Design review of the part shown in the three views and the two pictorial views. Dimensions are in mm from the part's minimum x, y and z. A direction names the side the tool comes from. Round coordinates to 2 decimals unless told otherwise and drop trailing zeros. Order: outer loops, then holes, each group sorted by start corner. A loop starts at its lowest first (then second) coordinate and runs counter-clockwise, first axis right, second up. Notation, with made-up numbers: M 27.5,15 L 35.5,15 A20 ccw 35.5,34 Z; hole C 84,-23 d7. An arc over 180 degrees is marked long. Write item = value, one per line. Start each with the question number.
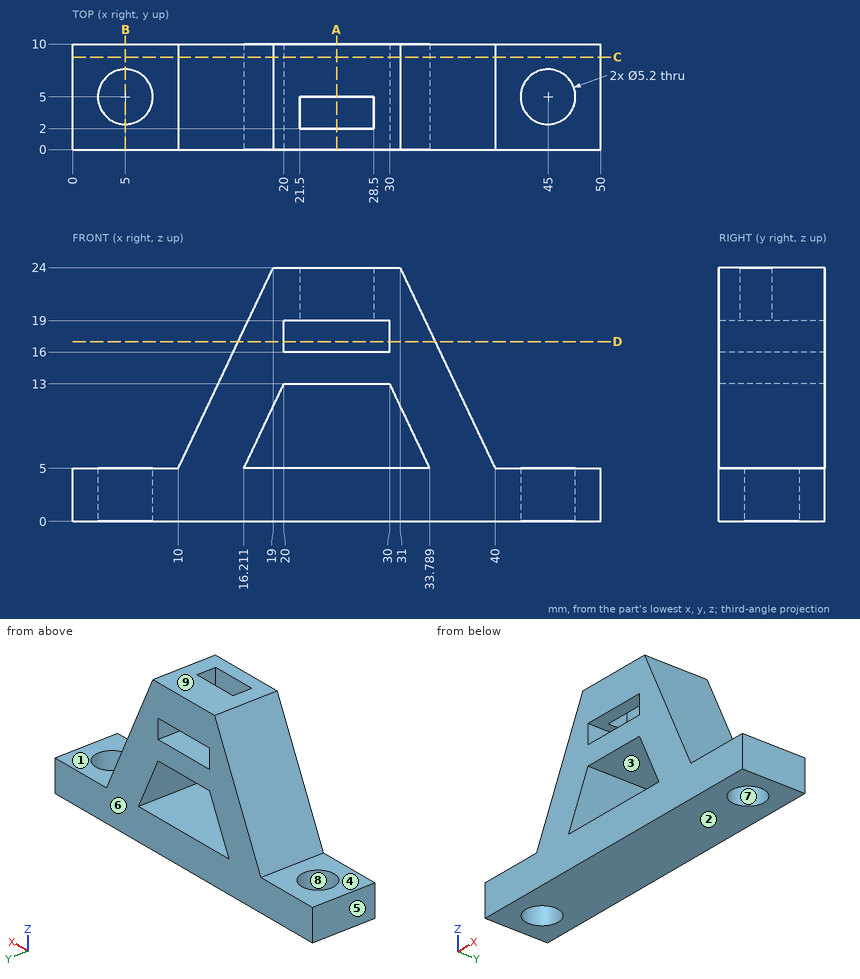
(1) Insertion check: pin 1 (1 mm diameter, centred on y = 3, z = 12.5, fed in from +X) (1 decimal); pin 2 (5 mm diameter, centred on x = 6, y = 5, fed in from +Z); pin 3 (1 mm diameter, centred on y = 4, z = 14.5, fed in from +X). Each pin has a flat end and moves straight along its axis. Give the tip position at first contact, or say it passes through.
(2) We need section C-C, the plane y = 8.75. Write out the cut boundary in (x, z).
(3) We need section B-B, the plane x = 5. Write out the cut boundary in (y, z).
(4) We need section D-D, the plane z = 17. Write out the cut boundary in (x, y) (1 decimal).
(5) We need section A-A, the plane x = 25. Write out the cut boundary in (y, z), then the cut area to 3 significant figures.
(6) Draft analysis for pull direction Y (two halves, no side actions). For the marked faces 6, 7, 8 and 9, state which applies: released by +Y, released by -Y, zero draft, split by the parting line, or undercut.
(7) For the marked faces 1, 2, 3, 4 and 5, list the 3-axis set-ups (+Z, -Z, +X, -X, +Y, -Y) from which the entire face can be reached by the end or side of a thin tool; tool diameter is ignored.
(8) For line 1 along Z through (x, y) = (21, 3.5); line 2 along Y through (x, z) = (5, 3.3); line 3 along Y through (x, z) = (23, 20), list the stretches that pass through material, from the lowest coordinate up.
Values:
q1.pin_1 = 36.7
q1.pin_2 = 5
q1.pin_3 = 35.74
q2.outline = M 0,0 L 50,0 L 50,5 L 40,5 L 31,24 L 19,24 L 10,5 L 0,5 Z; hole M 16.21,5 L 33.79,5 L 30,13 L 20,13 Z; hole M 20,16 L 30,16 L 30,19 L 20,19 Z
q3.outline = M 0,0 L 2.4,0 L 2.4,5 L 0,5 Z; M 7.6,0 L 10,0 L 10,5 L 7.6,5 Z
q4.outline = M 15.7,0 L 20,0 L 20,10 L 15.7,10 Z; M 30,0 L 34.3,0 L 34.3,10 L 30,10 Z
q5.outline = M 0,0 L 10,0 L 10,5 L 0,5 Z; M 0,13 L 10,13 L 10,16 L 0,16 Z; M 0,19 L 2,19 L 2,24 L 0,24 Z; M 5,19 L 10,19 L 10,24 L 5,24 Z
q5.area = 115 mm²
q6.face_6 = released by +Y
q6.face_7 = undercut
q6.face_8 = undercut
q6.face_9 = zero draft
q7.face_1 = +Z, +X, +Y, -Y
q7.face_2 = -Z, +X, -X, +Y, -Y
q7.face_3 = +Y, -Y
q7.face_4 = +Z, -X, +Y, -Y
q7.face_5 = +Z, -Z, -X, +Y, -Y
q8.line_1 = 0 to 5, 13 to 16, 19 to 24
q8.line_2 = 0 to 2.4, 7.6 to 10
q8.line_3 = 0 to 2, 5 to 10
